Could you check a few things on this model? Use its own coordinates, in mm. A direction names the side the tool comes from. Give positions to 0.01 mm unless a question says otherwise; leave off trailing zeros. Loops run counter-clockwise (first coordinate to the right, second up) from the corner with the lowest first, then second, coordinate; pieces in that order, holes last. Notation, with made-up numbers: (55.25, 68.5) - (78.25, 68.5) arc R15 ccw to (78.25, 95.5) - close; hole circle Ø9 at (28, 30.25). An arc over 180 degrees is marked (long way). Answer in a Markdown table with one row per item. Add a question column.
```python
from build123d import *

# Parameters (mm, degrees)
SKETCH2_W               = 79.375
SKETCH2_H               = 50.8
BOSS_EXTRUDE1_DEPTH     = 6.35
SKETCH3_W               = 66.675
SKETCH3_H               = 31.75
SKETCH3_W_2             = 25.4
SKETCH3_H_2             = 25.4
BOSS_EXTRUDE3_DEPTH     = 50.8
SKETCH4_W               = 25.4
SKETCH4_H               = 25.4
CUT_EXTRUDE4_DEPTH      = 7.35
CUT_EXTRUDE4_DEPTH_BACK = 58.15
SKETCH5_R               = 3.175
CUT_EXTRUDE5_DEPTH      = 42.275
SKETCH6_R               = 2.3876
CUT_EXTRUDE6_DEPTH      = 7.35
CIRPATTERN1_COUNT       = 4
CUT_EXTRUDE7_START      = -7.35
SKETCH7_R               = 2.3876
CUT_EXTRUDE7_DEPTH      = 65.5
SCALE1_SCALE            = 1.02


with BuildPart() as part:
    # Sketch2 → Boss-Extrude1 (new body)
    with BuildSketch(Plane(origin=(0, 0, 0), x_dir=(1, 0, 0), z_dir=(0, 1, 0))):
        Rectangle(SKETCH2_W, SKETCH2_H)
    boss_extrude1 = extrude(amount=BOSS_EXTRUDE1_DEPTH)

    # Sketch3 → Boss-Extrude3 (add)
    with BuildSketch(Plane(origin=(0, 6.35, 0), x_dir=(1, 0, 0), z_dir=(0, 1, 0))):
        with Locations((-3.175, 0)):
            Rectangle(SKETCH3_W, SKETCH3_H)
        with Locations((-20.6375, 0)):
            Rectangle(SKETCH3_W_2, SKETCH3_H_2, mode=Mode.SUBTRACT)
        with Locations((14.2875, 0)):
            Rectangle(SKETCH3_W_2, SKETCH3_H_2, mode=Mode.SUBTRACT)
    extrude(amount=BOSS_EXTRUDE3_DEPTH)

    # Mirror1: Boss-Extrude1 across plane
    add(boss_extrude1.mirror(Plane.ZX.offset(31.75)))

    # Sketch4 → Cut-Extrude4 (cut, two sides)
    with BuildSketch(Plane(origin=(0, 57.15, 0), x_dir=(1, 0, 0), z_dir=(0, 1, 0))) as cut_extrude4_sk:
        with Locations((-20.6375, 0)):
            Rectangle(SKETCH4_W, SKETCH4_H)
        with Locations((14.2875, 0)):
            Rectangle(SKETCH4_W, SKETCH4_H)
    extrude(amount=CUT_EXTRUDE4_DEPTH, mode=Mode.SUBTRACT)
    extrude(cut_extrude4_sk.sketch, amount=-CUT_EXTRUDE4_DEPTH_BACK, mode=Mode.SUBTRACT)

    # Sketch5 → Cut-Extrude5 (cut, through all)
    with BuildSketch(Plane.XY.offset(15.875)):
        with Locations((-20.6375, 31.75)):
            Circle(SKETCH5_R)
    extrude(amount=-CUT_EXTRUDE5_DEPTH, mode=Mode.SUBTRACT)

    # Sketch6 → Cut-Extrude6 (cut, through all)
    with BuildSketch(Plane(origin=(0, 6.35, 0), x_dir=(1, 0, 0), z_dir=(0, 1, 0))):
        with Locations((34.925, 0)):
            Circle(SKETCH6_R)
    cut_extrude6 = extrude(amount=-CUT_EXTRUDE6_DEPTH, mode=Mode.SUBTRACT)

    # CirPattern1: Cut-Extrude6 ×4 about axis, 1 skipped
    cirpattern1_axis = Axis((14.2875, 0, 0), (0, 1, 0))
    add([cut_extrude6.rotate(cirpattern1_axis, i * 360 / CIRPATTERN1_COUNT) for i in range(1, CIRPATTERN1_COUNT) if i not in (2,)], mode=Mode.SUBTRACT)

    # Sketch7 → Cut-Extrude7 (cut)
    with BuildSketch(Plane(origin=(0, 6.35, 0), x_dir=(1, 0, 0), z_dir=(0, 1, 0)).offset(CUT_EXTRUDE7_START)):
        with Locations((-20.6375, -20.6375)):
            Circle(SKETCH7_R)
    cut_extrude7 = extrude(amount=CUT_EXTRUDE7_DEPTH, mode=Mode.SUBTRACT)

    # Mirror2: Cut-Extrude7 across plane
    add(cut_extrude7.mirror(Plane.XY), mode=Mode.SUBTRACT)


with BuildPart() as part_1:
    # Scale1: scaled about (-0.988939035, 31.878583861, 0)
    add(part.part.scale(SCALE1_SCALE).moved(Location((0.019778781, -0.637571677, 0))))


solid = part_1.part
```
(1) For pin 1 Ø13 at (y, z) = (37, -6.5) entering from -X; pin 2 Ø3 at (y, z) = (36, -14.5) entering from +X; pin 3 Ø5 at (x, y) = (-17.5, 43.5) entering from -Z, each with a flat end and sliding along its axis, tell me the tip position at first contact or that it passes through.
(2) We'd pull the mould along Z, two halves only. Please class faces 6 (the cylindrical face through (-22.825, 2.556, 19.404)), 7 (the flat face through (30.786, 31, 0)), 8 (the flat face through (-15, 31, 12.954)), 9 (the flat face through (-4, 31, 16.192)): pulls with the +Z half, pulls with the -Z half, needs draft (parallel to the pull), parting line crosses it, or undercut.
(3) I want a section at B-B on x = 3.5. Please give me the cut outline in (y, z).
(4) I want a section at A-A on z = 12. Please give me the cut outline in (x, y).
(5) I want a section at D-D on z = 0. Please give me the cut outline in (x, y).
(6) I want a section at C-C on y = 9. Please give me the cut outline in (x, z).
(7) Please list where these lines run through material, in increasing order: line 1 (X direction, y = 31, z = 6); line 2 (X direction, y = 2.25, z = 0); line 3 (Z direction, x = -20.5, y = 45).
(8) On a 3-axis mill with a long thin cutter (end or side, diameter ignored), from which of +Z, -Z, +X, -X, +Y, -Y can I reach the whole of each face in a straight line? I mean faces 1 (the flat face through (-40.461, 3, 0)), 2 (the cylindrical face through (16.075, 2.646, -19.118)), 3 (the flat face through (-1, 61, -25.908)), 4 (the flat face through (1.639, 31, 0)), 5 (the flat face through (-4, 31, -16.192)). Say none if no direction works.
Reported:
| question | item | result |
|---|---|---|
| 1 | pin 1 | x = -37.22 |
| 1 | pin 2 | x = 30.79 |
| 1 | pin 3 | z = -16.19 |
| 2 | face 6 | undercut |
| 2 | face 7 | needs draft |
| 2 | face 8 | undercut |
| 2 | face 9 | pulls with the +Z half |
| 3 | outline | (-0.64, -25.91) - (5.84, -25.91) - (5.84, -16.19) - (57.66, -16.19) - (57.66, -25.91) - (64.13, -25.91) - (64.13, -12.95) - (-0.64, -12.95) - close; (-0.64, 12.95) - (64.13, 12.95) - (64.13, 25.91) - (57.66, 25.91) - (57.66, 16.19) - (5.84, 16.19) - (5.84, 25.91) - (-0.64, 25.91) - close |
| 4 | outline | (-40.46, -0.64) - (-33.98, -0.64) - (-33.98, 64.13) - (-40.46, 64.13) - (-40.46, 57.66) - (-37.22, 57.66) - (-37.22, 5.84) - (-40.46, 5.84) - close; (-8.08, -0.64) - (1.64, -0.64) - (1.64, 64.13) - (-8.08, 64.13) - close; (27.55, -0.64) - (40.5, -0.64) - (40.5, 5.84) - (30.79, 5.84) - (30.79, 57.66) - (40.5, 57.66) - (40.5, 64.13) - (27.55, 64.13) - close |
| 5 | outline | (-40.46, -0.64) - (-33.98, -0.64) - (-33.98, 64.13) - (-40.46, 64.13) - (-40.46, 57.66) - (-37.22, 57.66) - (-37.22, 5.84) - (-40.46, 5.84) - close; (-8.08, -0.64) - (1.64, -0.64) - (1.64, 64.13) - (-8.08, 64.13) - close; (27.55, -0.64) - (33.21, -0.64) - (33.21, 5.84) - (30.79, 5.84) - (30.79, 57.66) - (40.5, 57.66) - (40.5, 64.13) - (27.55, 64.13) - close; (38.08, -0.64) - (40.5, -0.64) - (40.5, 5.84) - (38.08, 5.84) - close |
| 6 | outline | (-37.22, -16.19) - (30.79, -16.19) - (30.79, 16.19) - (-37.22, 16.19) - close; hole (-33.98, -12.95) - (-8.08, -12.95) - (-8.08, 12.95) - (-33.98, 12.95) - close; hole (1.64, -12.95) - (27.55, -12.95) - (27.55, 12.95) - (1.64, 12.95) - close |
| 7 | line 1 | -37.22 to -33.98, -8.08 to 1.64, 27.55 to 30.79 |
| 7 | line 2 | -40.46 to -33.98, -8.08 to 1.64, 27.55 to 33.21, 38.08 to 40.5 |
| 7 | line 3 | -16.19 to -12.95, 12.95 to 16.19 |
| 8 | face 1 | +Z, -Z, -X, +Y, -Y |
| 8 | face 2 | -Y |
| 8 | face 3 | -Z, +X, -X, +Y, -Y |
| 8 | face 4 | +Y, -Y |
| 8 | face 5 | -Z, +X, -X |
